Can you work these out from the drawing? Everything is in mm from the part's minimum corner. A direction names the side the tool comes from. Coordinates: 2 decimals unless noted, no trailing zeros. Order: outer loops, then holes, each group sorted by start corner. A loop starts at its lowest first (then second) coordinate and runs counter-clockwise, first axis right, second up. Notation, with made-up numbers: (60, 47.5) -> (90, 47.5) arc R36 cw to (90, 81.5) -> close; hole circle Ø2 at (33.5, 11.25). An arc over 180 degrees is marked (long way). Use a Markdown table: item, result. Add a question column.
1) If we section it at A-A (z = 6): Write out the boundary of the cut face in (x, y).
2) If we section it at C-C (y = 3.25): Write out the boundary of the cut face in (x, z).
3) If I drill on L1, parallel to Y at x = 17, z = 11.5; L2, parallel to Z at x = 8.25, y = 7.5, over which ranges is the centre line in solid material (lowest first)? Write a range as [from, to].
4) Will these pins go through, and if not, where does the flat tip stop? pin 1 Ø1 at (y, z) = (7.5, 8.5) entering from +X; pin 2 Ø2 at (y, z) = (10, 13.5) entering from +X; pin 3 Ø1 at (y, z) = (8.5, 8) entering from -X; pin 4 Ø10 at (x, y) = (12.5, 3.5) entering from +Z.
5) If we section it at D-D (x = 11.5): Write out the boundary of the cut face in (y, z), plus the area to 3 significant figures.
6) Which directions (+Z, -Z, +X, -X, +Y, -Y) give clear straight access to the entire face, cutting with the end or side of a thin tool? Please do the marked faces 1 and 2.
7) If we section it at B-B (x = 6): Write out the boundary of the cut face in (y, z), plus the area to 3 significant figures.
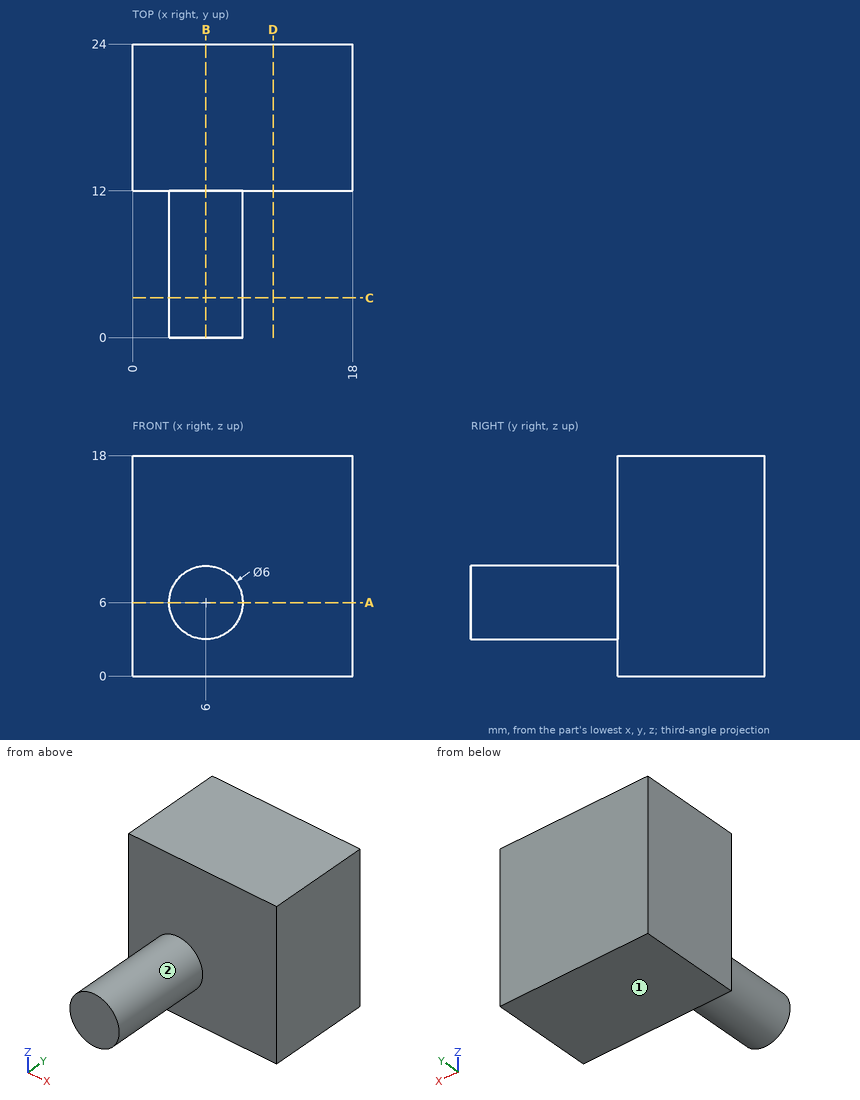
Answer sheet:
| question | item | result |
|---|---|---|
| 1 | outline | (0, 12) -> (3, 12) -> (3, 0) -> (9, 0) -> (9, 12) -> (18, 12) -> (18, 24) -> (0, 24) -> close |
| 2 | outline | circle Ø6 at (6, 6) |
| 3 | L1 | [12, 24] |
| 3 | L2 | [4.02, 7.98] |
| 4 | pin 1 | x = 8.24 |
| 4 | pin 2 | through |
| 4 | pin 3 | x = 3.4 |
| 4 | pin 4 | z = 8.6 |
| 5 | outline | (12, 0) -> (24, 0) -> (24, 18) -> (12, 18) -> close |
| 5 | area | 216 mm2 |
| 6 | face 1 | -Z, +X, -X, +Y, -Y |
| 6 | face 2 | -Y |
| 7 | outline | (0, 3) -> (12, 3) -> (12, 0) -> (24, 0) -> (24, 18) -> (12, 18) -> (12, 9) -> (0, 9) -> close |
| 7 | area | 288 mm2 |
